Here's how the part is built. I have some questions about the finished solid (model axes, mm). Face numbers are marked on the shaded views. Round coordinates to 2 decimals unless told otherwise and drop trailing zeros. Order: outer loops, then holes, each group sorted by start corner. A loop starts at its lowest first (then second) coordinate and runs counter-clockwise, first axis right, second up. Notation, with made-up numbers: (-37.5, 3.25) -> (3.5, 3.25) arc R17 ccw to (3.5, 16.25) -> close; hole circle Ø7 at (77.25, 66). An arc over 180 degrees is marked (long way). One line per item, written item: value.
```python
from build123d import *

# Parameters (mm, degrees)
SKETCH1_W           = 62.15
SKETCH1_H           = 62.15
BOSS_EXTRUDE1_DEPTH = 5
CUT_EXTRUDE1_REACH  = 46.23
SKETCH2_R           = 1.5
SKETCH3_R           = 28.575
SKETCH3_R_2         = 26.075
BOSS_EXTRUDE2_DEPTH = 2.5
CUT_EXTRUDE2_REACH  = 46.23
SKETCH4_R           = 15.875
SKETCH5_R           = 3
CUT_EXTRUDE3_DEPTH  = 2


with BuildPart() as part:
    # Sketch1 → Boss-Extrude1 (new body)
    with BuildSketch(Plane(origin=(0, 0, 0), x_dir=(1, 0, 0), z_dir=(0, 1, 0))):
        Rectangle(SKETCH1_W, SKETCH1_H)
    extrude(amount=BOSS_EXTRUDE1_DEPTH)

    # Sketch2 → Cut-Extrude1 (cut, up to next)
    with BuildSketch(Plane(origin=(0, 5, 0), x_dir=(1, 0, 0), z_dir=(0, 1, 0)), mode=Mode.PRIVATE) as cut_extrude1_sk1:
        with Locations(Location((-26.075, 26.075, 0), (0, 0, 270))):
            Circle(SKETCH2_R)
    cut_extrude1_tool1 = extrude(cut_extrude1_sk1.sketch, amount=-CUT_EXTRUDE1_REACH, mode=Mode.PRIVATE) & part.part
    # Sketch2 → Cut-Extrude1 (cut, up to next)
    with BuildSketch(Plane(origin=(0, 5, 0), x_dir=(1, 0, 0), z_dir=(0, 1, 0)), mode=Mode.PRIVATE) as cut_extrude1_sk2:
        with Locations(Location((-26.075, -26.075, 0), (0, 0, 270))):
            Circle(SKETCH2_R)
    cut_extrude1_tool2 = extrude(cut_extrude1_sk2.sketch, amount=-CUT_EXTRUDE1_REACH, mode=Mode.PRIVATE) & part.part
    # Sketch2 → Cut-Extrude1 (cut, up to next)
    with BuildSketch(Plane(origin=(0, 5, 0), x_dir=(1, 0, 0), z_dir=(0, 1, 0)), mode=Mode.PRIVATE) as cut_extrude1_sk3:
        with Locations(Location((26.075, -26.075, 0), (0, 0, 270))):
            Circle(SKETCH2_R)
    cut_extrude1_tool3 = extrude(cut_extrude1_sk3.sketch, amount=-CUT_EXTRUDE1_REACH, mode=Mode.PRIVATE) & part.part
    # Sketch2 → Cut-Extrude1 (cut, up to next)
    with BuildSketch(Plane(origin=(0, 5, 0), x_dir=(1, 0, 0), z_dir=(0, 1, 0)), mode=Mode.PRIVATE) as cut_extrude1_sk4:
        with Locations(Location((26.075, 26.075, 0), (0, 0, 270))):
            Circle(SKETCH2_R)
    cut_extrude1_tool4 = extrude(cut_extrude1_sk4.sketch, amount=-CUT_EXTRUDE1_REACH, mode=Mode.PRIVATE) & part.part
    add(cut_extrude1_tool1.solids().sort_by_distance((-26.075, 5, -26.075))[0], mode=Mode.SUBTRACT)
    add(cut_extrude1_tool2.solids().sort_by_distance((-26.075, 5, 26.075))[0], mode=Mode.SUBTRACT)
    add(cut_extrude1_tool3.solids().sort_by_distance((26.075, 5, 26.075))[0], mode=Mode.SUBTRACT)
    add(cut_extrude1_tool4.solids().sort_by_distance((26.075, 5, -26.075))[0], mode=Mode.SUBTRACT)

    # Sketch3 → Boss-Extrude2 (add)
    with BuildSketch(Plane(origin=(0, 5, 0), x_dir=(1, 0, 0), z_dir=(0, 1, 0))):
        with Locations(Location((0, 0, 0), (0, 0, 270))):
            Circle(SKETCH3_R)
        with Locations(Location((0, 0, 0), (0, 0, 270))):
            Circle(SKETCH3_R_2, mode=Mode.SUBTRACT)
    extrude(amount=BOSS_EXTRUDE2_DEPTH)

    # Sketch4 → Cut-Extrude2 (cut, up to next)
    with BuildSketch(Plane(origin=(0, 5, 0), x_dir=(1, 0, 0), z_dir=(0, 1, 0)), mode=Mode.PRIVATE) as cut_extrude2_sk1:
        with Locations(Location((0, 0, 0), (0, 0, 270))):
            Circle(SKETCH4_R)
    cut_extrude2_tool1 = extrude(cut_extrude2_sk1.sketch, amount=-CUT_EXTRUDE2_REACH, mode=Mode.PRIVATE) & part.part
    add(cut_extrude2_tool1.solids().sort_by_distance((0, 5, 0))[0], mode=Mode.SUBTRACT)

    # Sketch5 → Cut-Extrude3 (cut)
    with BuildSketch(Plane.XZ):
        with Locations(Location((-26.075, 26.075, 0), (0, 0, 270))):
            Circle(SKETCH5_R)
        with Locations(Location((-26.075, -26.075, 0), (0, 0, 90))):
            Circle(SKETCH5_R)
        with Locations(Location((26.075, -26.075, 0), (0, 0, 270))):
            Circle(SKETCH5_R)
        with Locations(Location((26.075, 26.075, 0), (0, 0, 90))):
            Circle(SKETCH5_R)
    extrude(amount=-CUT_EXTRUDE3_DEPTH, mode=Mode.SUBTRACT)


solid = part.part
```
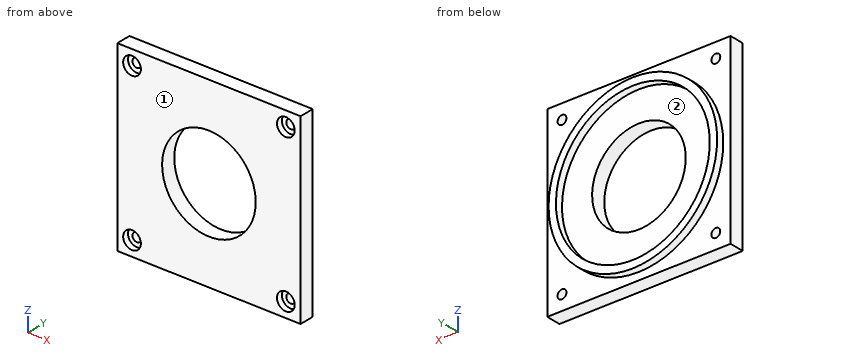
Q1. For P1, Ø5, axis at x = -26.075, z = 26.075, coming from the +Y side; P2, Ø5, axis at x = 26.075, z = 26.075, coming from the -Y side; P3, Ø2, axis at x = -0.5, y = 6.5, coming from the -Z side (3 decimals), each with a flat end and sliding along its axis, tell me the tip position at first contact or that it passes through.
Answers:
P1: y = 5
P2: y = 2
P3: z = -28.575
Q2. If we mould it in two halves opening along Z, with no side actions, what happens to the marked faces 1 and 2? For each: pulls with the +Z half, pulls with the -Z half, needs draft (parallel to the pull), parting line crosses it, or undercut.
Answers:
face 1: needs draft
face 2: undercut
Q3. I want a section at A-A on z = 0. Write out the boundary of the cut face in (x, y) (3 decimals), then the cut area to 4 significant figures.
Answers:
outline: (-31.075, 0) -> (-15.875, 0) -> (-15.875, 5) -> (-26.075, 5) -> (-26.075, 7.5) -> (-28.575, 7.5) -> (-28.575, 5) -> (-31.075, 5) -> close; (15.875, 0) -> (31.075, 0) -> (31.075, 5) -> (28.575, 5) -> (28.575, 7.5) -> (26.075, 7.5) -> (26.075, 5) -> (15.875, 5) -> close
area: 164.5 mm2
Q4. I want a section at C-C on y = 3.5. Write out the boundary of the cut face in (x, z) (3 decimals).
Answers:
outline: (-31.075, -31.075) -> (31.075, -31.075) -> (31.075, 31.075) -> (-31.075, 31.075) -> close; hole circle Ø3 at (-26.075, -26.075); hole circle Ø3 at (-26.075, 26.075); hole circle Ø31.75 at (0, 0); hole circle Ø3 at (26.075, -26.075); hole circle Ø3 at (26.075, 26.075)
Q5. I want a section at B-B on x = 0. Write out the boundary of the cut face in (y, z) (3 decimals), then the cut area to 4 significant figures.
Answers:
outline: (0, -31.075) -> (5, -31.075) -> (5, -28.575) -> (7.5, -28.575) -> (7.5, -26.075) -> (5, -26.075) -> (5, -15.875) -> (0, -15.875) -> close; (0, 15.875) -> (5, 15.875) -> (5, 26.075) -> (7.5, 26.075) -> (7.5, 28.575) -> (5, 28.575) -> (5, 31.075) -> (0, 31.075) -> close
area: 164.5 mm2
Q6. I need wall thicknesses on line 1 along X through (y, z) = (1.5, 24) (3 decimals); line 2 along Z through (x, y) = (25, 3) (3 decimals); line 3 along X through (y, z) = (4, 27) (3 decimals). Which ranges of each line are inside material? Lowest first, please.
Answers:
line 1: -31.075 to -28.242, -23.908 to 23.908, 28.242 to 31.075
line 2: -31.075 to -27.121, -25.029 to 25.029, 27.121 to 31.075
line 3: -31.075 to -27.256, -24.894 to 24.894, 27.256 to 31.075
Q7. I want a section at D-D on z = 17. Write out the boundary of the cut face in (x, y) (3 decimals).
Answers:
outline: (-31.075, 0) -> (31.075, 0) -> (31.075, 5) -> (22.968, 5) -> (22.968, 7.5) -> (19.771, 7.5) -> (19.771, 5) -> (-19.771, 5) -> (-19.771, 7.5) -> (-22.968, 7.5) -> (-22.968, 5) -> (-31.075, 5) -> close
